```python
from build123d import *

# Parameters (mm, degrees)
BOSS_EXTRUDE1_DEPTH = 6.4516
SKETCH2_W           = 19.05
SKETCH2_H           = 4.826
BOSS_EXTRUDE2_DEPTH = 10.16
FILLET1_R           = 5.08
FILLET2_R           = 0.762
SKETCH4_W           = 6.4262
SKETCH4_H           = 12.5476
CUT_EXTRUDE1_DEPTH  = 0.508
BOSS_EXTRUDE3_DEPTH = 3.0861
CHAMFER1_SIZE       = 2.794
CUT_EXTRUDE2_DEPTH  = 3.556


with BuildPart() as part:
    # Sketch1 → Boss-Extrude1 (new body)
    with BuildSketch(Plane(origin=(0, 0, 0), x_dir=(1, 0, 0), z_dir=(0, 1, 0))):
        Polygon((-3.0988, -12.8524), (-3.0988, -25.4), (9.525, -25.4), (9.525, 25.4), (-9.525, 25.4), (-9.525, -12.8524), align=None)
    extrude(amount=BOSS_EXTRUDE1_DEPTH)

    # Sketch2 → Boss-Extrude2 (add)
    with BuildSketch(Plane(origin=(0, 6.4516, 0), x_dir=(1, 0, 0), z_dir=(0, 1, 0))):
        with Locations((0, 22.987)):
            Rectangle(SKETCH2_W, SKETCH2_H)
    extrude(amount=BOSS_EXTRUDE2_DEPTH)

    # Fillet1
    fillet1_edges = [part.edges().sort_by_distance(p)[0] for p in [
        (0, 6.4516, -20.574),
    ]]
    fillet(fillet1_edges, radius=FILLET1_R)

    # Fillet2
    fillet2_edges = [part.edges().sort_by_distance(p)[0] for p in [
        (0, 16.6116, -20.574),
        (0, 16.6116, -25.4),
    ]]
    fillet(fillet2_edges, radius=FILLET2_R)

    # Sketch4 → Cut-Extrude1 (cut)
    with BuildSketch(Plane(origin=(0, 6.4516, 0), x_dir=(1, 0, 0), z_dir=(0, 1, 0))):
        with Locations((6.3119, -19.1262)):
            Rectangle(SKETCH4_W, SKETCH4_H)
    extrude(amount=-CUT_EXTRUDE1_DEPTH, mode=Mode.SUBTRACT)

    # Sketch5 → Boss-Extrude3 (add, symmetric)
    with BuildSketch(Plane(origin=(0, 0, 0), x_dir=(0, 0, -1), z_dir=(1, 0, 0))):
        Polygon((-25.4, 6.4516), (-12.8524, 6.4516), (-24.511, 9.96315), (-25.4, 9.96315), align=None)
        Polygon((-25.4, 0), (-25.4, -3.51155), (-12.8524, 0), align=None)
    extrude(amount=BOSS_EXTRUDE3_DEPTH, both=True)

    # Chamfer1
    chamfer1_edges = [part.edges().sort_by_distance(p)[0] for p in [
        (0, 0, -25.4),
    ]]
    chamfer(chamfer1_edges, length=CHAMFER1_SIZE)

    # Sketch6 → Cut-Extrude2 (cut)
    with BuildSketch(Plane.XZ):
        Polygon((3.175, 23.851678881), (7.239, 23.851678881), (7.239, -21.9964), (-7.239, -21.9964), (-7.239, 10.702998039), (-3.175, 10.702998039), (-3.175, 1.273136021), (3.175, 1.273136021), align=None)
    extrude(amount=-CUT_EXTRUDE2_DEPTH, mode=Mode.SUBTRACT)


solid = part.part
```
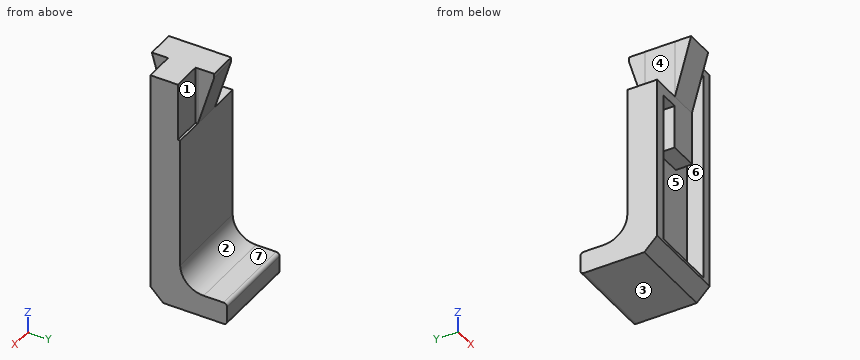
Here's how the part is built. I have some questions about the finished solid (model axes, mm). Face numbers are marked on the shaded views. A direction names the side the tool comes from. Coordinates: 2 decimals unless noted, no trailing zeros. Order: outer loops, then holes, each group sorted by start corner. A loop starts at its lowest first (then second) coordinate and runs counter-clockwise, first axis right, second up.
Item 1: If we section it at D-D, the plane z = -9.5: List the corners of the cut face in (x, y) for me (3 decimals), then the cut area to 3 significant figures.
Response values:
outline: (-9.525, 0) - (-7.239, 0) - (-7.239, 3.556) - (7.239, 3.556) - (7.239, 0) - (9.525, 0) - (9.525, 6.452) - (-9.525, 6.452) - close
area: 71.4 mm2
Item 2: If we section it at C-C, the plane y = 5: List the corners of the cut face in (x, z) for me (3 decimals), then the cut area to 3 significant figures.
Response values:
outline: (-9.525, -25.4) - (9.525, -25.4) - (9.525, 25.4) - (-3.099, 25.4) - (-3.099, 12.852) - (-9.525, 12.852) - close
area: 887 mm2
Item 3: If we section it at A-A, the plane x = -5.75: List the corners of the cut face in (y, z) for me, then the cut area to 3 significant figures.
Response values:
outline: (0, -22.61) - (2.79, -25.4) - (15.85, -25.4) arc R0.76 ccw to (16.61, -24.64) - (16.61, -21.34) arc R0.76 ccw to (15.85, -20.57) - (11.53, -20.57) arc R5.08 cw to (6.45, -15.49) - (6.45, 12.85) - (0, 12.85) - (0, 10.7) - (3.56, 10.7) - (3.56, -22) - (0, -22) - close
area: 181 mm2
Item 4: Thinking about a two-plate mould opening in X: for the marked faces 4, 5, 6 and 7, which applies, pulls with the +X half, pulls with the -X half, needs draft (parallel to the pull), parting line crosses it, or undercut?
Response values:
face 4: pulls with the -X half
face 5: undercut
face 6: undercut
face 7: needs draft
Item 5: Which directions (+Z, -Z, +X, -X, +Y, -Y) give clear straight access to the entire face, cutting with the end or side of a thin tool? Please do the marked faces 1, 2 and 3.
Response values:
face 1: +Z, +X, +Y
face 2: +X, -X, +Y
face 3: -Z, +X, -X, +Y, -Y
Item 6: If we section it at B-B, the plane y = 9: List the corners of the cut face in (x, z) for me (3 decimals).
Response values:
outline: (-9.525, -25.4) - (9.525, -25.4) - (9.525, -19.898) - (-9.525, -19.898) - close; (-3.086, 21.313) - (3.086, 21.313) - (3.086, 25.4) - (-3.086, 25.4) - close
Item 7: I'm going to push flat-ended pins straight in: pin 1 Ø6 at (x, z) = (4.5, -2) entering from +Y; pin 2 Ø1.9 at (y, z) = (1.5, 18.5) entering from -X; pin 3 Ø7 at (x, z) = (7, 21) entering from +Y. Where does each tip first touch, or does it pass through?
Response values:
pin 1: stops at y = 6.45
pin 2: stops at x = -3.1
pin 3: stops at y = 5.94
Item 8: I need wall thicknesses on probe 1 along X at (y, z) = (2.75, -19.5) (3 decimals); probe 2 along Y at (x, z) = (2.75, -11); probe 3 along Z at (x, y) = (1, 14). Which ranges of each line are inside material? Lowest first, please.
Response values:
probe 1: x = -9.525 to -7.239, 7.239 to 9.525
probe 2: y = 3.56 to 6.45
probe 3: z = -25.4 to -20.57
